Verification items for the finished model (mm, model axes). A direction names the side the tool comes from. Coordinates: 2 decimals unless noted, no trailing zeros. Write each loop counter-clockwise with the first axis right and the second up, starting at its lowest first coordinate (ties: lowest second). Pieces come first, ordered by that corner, then holes. Notation, with made-up numbers: (68.5, 68) - (86.5, 68) arc R18 ccw to (86.5, 98) - close; hole circle Ø8 at (3, -26.75). An arc over 180 degrees is marked (long way). Use one line per item in the form item = value. Start each with the question number.
(1) Sectioned sample at B-B (z = -75.5). Record the cut outline in (x, y).
(2) Material ranges on line 1 (Y direction, x = -20, z = -208.5); line 2 (Z direction, x = -16, y = -9); line 3 (X direction, y = 50.5, z = -106.5), recorded low to high. Write a range as [from, to].
(3) Tool access check on faces 1 (the flat face through (0, -49, -97)), 2 (the flat face through (0, -49, -47)), 3 (the flat face through (25, -49, -72)), 4 (the flat face through (36.832, 29.087, -114.236)), 5 (the flat face through (-25, -49, -72)). Record the directions out of +Z, -Z, +X, -X, +Y, -Y that give a thin tool (end or side, any length) a straight path to the whole face; none if there is none.
(4) Sectioned sample at C-C (y = 37.5). Record the cut outline in (x, z), and give its area (3 significant figures).
(5) Sectioned sample at D-D (x = 37.5). Record the cut outline in (y, z).
(6) Sectioned sample at A-A (x = 2). Record the cut outline in (y, z), and give its area (3 significant figures).
(7) Gauge pin test, flat ends, axial feed: pin 1 Ø1 at (x, y) = (23.5, -23) entering from +Z; pin 2 Ø15 at (y, z) = (-64.5, -68.5) entering from +X; pin 3 Ø10 at (x, z) = (-19.5, -148.5) entering from -Y. Record the tip position at first contact, or that the pin passes through.
from build123d import *

# Parameters (mm, degrees)
BOSS_EXTRUDE1_DEPTH = 59
SKETCH3_W           = 50
SKETCH3_H           = 50
BOSS_EXTRUDE2_DEPTH = 100


with BuildPart() as part:
    # Sketch1 → Boss-Extrude1 (new body)
    with BuildSketch(Plane(origin=(0, 0, 0), x_dir=(1, 0, 0), z_dir=(0, 1, 0))):
        Polygon((-25, -10), (25, -10), (49, 242), (-49, 242), align=None)
    extrude(amount=BOSS_EXTRUDE1_DEPTH)

    # Sketch3 → Boss-Extrude2 (add)
    with BuildSketch(Plane(origin=(0, 0, 0), x_dir=(1, 0, 0), z_dir=(0, 1, 0))):
        with Locations((0, 72)):
            Rectangle(SKETCH3_W, SKETCH3_H)
    extrude(amount=-BOSS_EXTRUDE2_DEPTH)


solid = part.part
Answers below:
q1.outline = (-33.14, 0) - (-25, 0) - (-25, -100) - (25, -100) - (25, 0) - (33.14, 0) - (33.14, 59) - (-33.14, 59) - close
q2.line_1 = [0, 59]
q2.line_2 = [-97, -47]
q2.line_3 = [-36.1, 36.1]
q3.face_1 = -Z, +X, -X, -Y
q3.face_2 = +Z, +X, -X, -Y
q3.face_3 = +Z, -Z, +X, -Y
q3.face_4 = +Z, +X, +Y, -Y
q3.face_5 = +Z, -Z, -X, -Y
q4.outline = (-49, -242) - (49, -242) - (25, 10) - (-25, 10) - close
q4.area = 18,600 mm2
q5.outline = (0, -242) - (59, -242) - (59, -121.25) - (0, -121.25) - close
q6.outline = (-100, -97) - (0, -97) - (0, -242) - (59, -242) - (59, 10) - (0, 10) - (0, -47) - (-100, -47) - close
q6.area = 19,900 mm2
q7.pin_1 = -47
q7.pin_2 = 25
q7.pin_3 = 0
